For this review, take the finished solid that the model builds, in its own axes (mm). Face numbers are marked on the shaded views. A direction names the side the tool comes from. Give positions to 0.01 mm unless a question says otherwise; leave off trailing zeros. Order: outer loops, then holes, each group sorted by start corner. A loop starts at its lowest first (then second) coordinate and runs counter-clockwise, first axis right, second up. Notation, with made-up numbers: (33, 55.25) - (89, 55.25) arc R33 cw to (89, 89.25) - close; hole circle Ø9 at (-1.5, 80). An arc over 180 degrees is marked (long way). Answer as a JSON object with one key per item and string values. Group by question number.
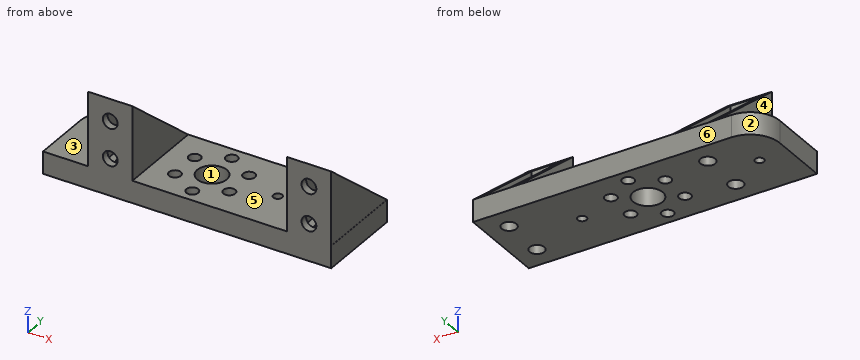
from build123d import *

# Parameters (mm, degrees)
SKETCH1_R           = 2
SKETCH1_R_2         = 0.6
SKETCH1_R_3         = 1
BOSS_EXTRUDE1_DEPTH = 3
SKETCH3_R           = 0.8
CUT_EXTRUDE1_DEPTH  = 3
CIRPATTERN1_COUNT   = 6
BOSS_EXTRUDE3_DEPTH = 10
CUT_EXTRUDE2_DEPTH  = 45
SKETCH7_R           = 1
CUT_EXTRUDE3_DEPTH  = 10
LPATTERN1_COUNT     = 2
LPATTERN1_PITCH     = 26.886757186


with BuildPart() as part:
    # Sketch1 → Boss-Extrude1 (new body)
    with BuildSketch(Plane.XY):
        with BuildLine():
            Line((-23.1, -6), (15.9, -6))
            Line((15.9, -6), (15.9, 6))
            Line((15.9, 6), (-19.1, 6))
            ThreePointArc((-19.1, 6), (-21.928427125, 4.828427125), (-23.1, 2))
            Line((-23.1, 2), (-23.1, -6))
        make_face()
        with Locations((-4, 0)):
            Circle(SKETCH1_R, mode=Mode.SUBTRACT)
        with Locations((4.9, 0)):
            Circle(SKETCH1_R_2, mode=Mode.SUBTRACT)
        with Locations((-19.1, 0)):
            Circle(SKETCH1_R_2, mode=Mode.SUBTRACT)
        with Locations((12.9, 3)):
            Circle(SKETCH1_R_3, mode=Mode.SUBTRACT)
        with Locations((12.9, -3)):
            Circle(SKETCH1_R_3, mode=Mode.SUBTRACT)
        with Locations((-14, -3)):
            Circle(SKETCH1_R_3, mode=Mode.SUBTRACT)
        with Locations((-14, 3)):
            Circle(SKETCH1_R_3, mode=Mode.SUBTRACT)
    extrude(amount=BOSS_EXTRUDE1_DEPTH)

    # Sketch3 → Cut-Extrude1 (cut)
    with BuildSketch(Plane.XY.offset(3)):
        with Locations((-4, 4.25)):
            Circle(SKETCH3_R)
    cut_extrude1 = extrude(amount=-CUT_EXTRUDE1_DEPTH, mode=Mode.SUBTRACT)

    # CirPattern1: Cut-Extrude1 ×6 about axis
    cirpattern1_axis = Axis((-4, 0, 0), (0, 0, 1))
    for i in range(1, CIRPATTERN1_COUNT):
        add(cut_extrude1.rotate(cirpattern1_axis, i * 360 / CIRPATTERN1_COUNT), mode=Mode.SUBTRACT)

    # Sketch4 → Boss-Extrude3 (add)
    with BuildSketch(Plane.XY.offset(3)):
        Polygon((-17, 6), (-17, -6), (-11, -6), (-11, 6), (-12, 6), (-12, -5), (-16, -5), (-16, 6), align=None)
    boss_extrude3 = extrude(amount=BOSS_EXTRUDE3_DEPTH)

    # Sketch5 → Cut-Extrude2 (cut)
    with BuildSketch(Plane.ZY.offset(17)):
        Polygon((3, 6), (13, -6), (13, 6), align=None)
    cut_extrude2 = extrude(amount=-CUT_EXTRUDE2_DEPTH, mode=Mode.SUBTRACT)

    # Sketch7 → Cut-Extrude3 (cut)
    with BuildSketch(Plane(origin=(0, -5, 0), x_dir=(1, 0, 0), z_dir=(0, 1, 0))):
        with Locations((-14, -5)):
            Circle(SKETCH7_R)
        with Locations((-14, -10)):
            Circle(SKETCH7_R)
    cut_extrude3 = extrude(amount=-CUT_EXTRUDE3_DEPTH, mode=Mode.SUBTRACT)

    # LPattern1: Boss-Extrude3, Cut-Extrude2, Cut-Extrude3 ×2
    with Locations(*[(i * LPATTERN1_PITCH, 0, 0) for i in range(1, LPATTERN1_COUNT)]):
        add(boss_extrude3)
        add(cut_extrude2, mode=Mode.SUBTRACT)
        add(cut_extrude3, mode=Mode.SUBTRACT)


solid = part.part
1) For pin 1 (1.2 mm diameter, centred on x = -14, z = 10, fed in from -Y); pin 2 (2.5 mm diameter, centred on x = -7.68, y = 2.13, fed in from +Z); pin 3 (4.5 mm diameter, centred on y = 1, z = 5.5, fed in from +X); pin 4 (1.2 mm diameter, centred on x = 13, z = 6, fed in from +Y), all flat-tipped, find the tip position at first contact; note any pin that passes through.
2) Consider section A-A (y = 0). Give the number of separate pieces and of enclosed holes in the cut face, plus the area to 3 significant figures.
3) Consider section D-D (z = 10). Give the boundary of the cut face in (x, y), plus the area to 3 significant figures.
4) For line 1 (Y direction, x = 12.9, z = 1.1); line 2 (X direction, y = 1, z = 7); line 3 (Y direction, x = -4, z = 1.6), list the stretches that pass through material, from the lowest coordinate up.
5) For the marked faces 4, 5 and 6, list the 3-axis set-ups (+Z, -Z, +X, -X, +Y, -Y) from which the entire face can be reached by the end or side of a thin tool; tool diameter is ignored.
6) Mouldability with a two-part tool opening along Y and no side actions: class the marked faces 1, 2 and 3 as released by +Y, released by -Y, zero draft, split by the parting line, or undercut.
7) Consider section B-B (z = 3.5). Give the boundary of the cut face in (x, y).
8) Consider section C-C (x = -14). Give the boundary of the cut face in (y, z).
Result set:
{
 "1": {"pin 1": "passes through", "pin 2": "stops at z = 3", "pin 3": "stops at x = 15.89", "pin 4": "stops at y = -5"},
 "2": {"separate pieces": "4", "enclosed holes": "0", "area": "118 mm2"},
 "3": {"outline": "(-17, -6) - (-15, -6) - (-15, -5) - (-16, -5) - (-16, -2.4) - (-17, -2.4) - close; (-13, -6) - (-11, -6) - (-11, -2.4) - (-12, -2.4) - (-12, -5) - (-13, -5) - close; (9.89, -6) - (11.89, -6) - (11.89, -5) - (10.89, -5) - (10.89, -2.4) - (9.89, -2.4) - close; (13.89, -6) - (15.89, -6) - (15.89, -2.4) - (14.89, -2.4) - (14.89, -5) - (13.89, -5) - close", "area": "18.4 mm2"},
 "4": {"line 1": "y = -6 to -4, -2 to 2, 4 to 6", "line 2": "x = -17 to -16, -12 to -11, 9.89 to 10.89, 14.89 to 15.89", "line 3": "y = -6 to -5.05, -3.45 to -2, 2 to 3.45, 5.05 to 6"},
 "5": {"face 4": "+Z, -X, +Y, -Y", "face 5": "+Z, +Y, -Y", "face 6": "+Z, -Z, +X, -X, +Y"},
 "6": {"face 1": "undercut", "face 2": "released by +Y", "face 3": "zero draft"},
 "7": {"outline": "(-17, -6) - (-11, -6) - (-11, 5.4) - (-12, 5.4) - (-12, -5) - (-16, -5) - (-16, 5.4) - (-17, 5.4) - close; (9.89, -6) - (15.89, -6) - (15.89, 5.4) - (14.89, 5.4) - (14.89, -5) - (10.89, -5) - (10.89, 5.4) - (9.89, 5.4) - close"},
 "8": {"outline": "(-6, 0) - (-4, 0) - (-4, 3) - (-5, 3) - (-5, 4) - (-6, 4) - close; (-6, 6) - (-5, 6) - (-5, 9) - (-6, 9) - close; (-6, 11) - (-5, 11) - (-5, 12.17) - (-6, 13) - close; (-2, 0) - (2, 0) - (2, 3) - (-2, 3) - close; (4, 0) - (6, 0) - (6, 3) - (4, 3) - close"}
}
